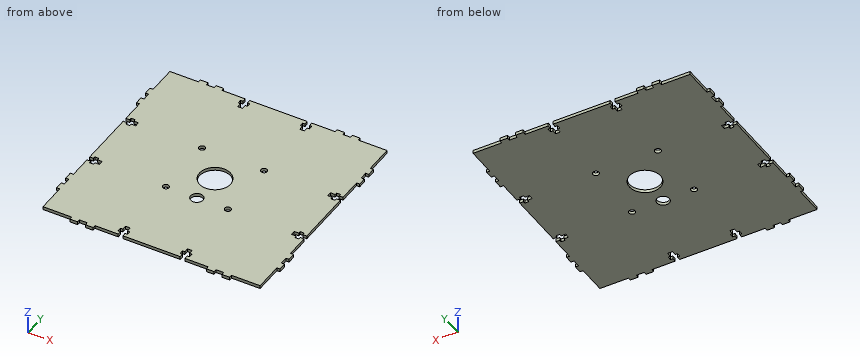
```python
from build123d import *

# Parameters (mm, degrees)
SKETCH_1_R      = 10
SKETCH_1_R_2    = 4
SKETCH_1_R_3    = 2
EXTRUDE_1_DEPTH = 2


with BuildPart() as part:
    # 草图1 → 凸台-拉伸1 (new body)
    with BuildSketch(Plane.XY):
        Polygon((317.453360513, 257.462931603), (317.453360513, 258.962931603), (314.853360513, 258.962931603), (314.853360513, 257.462931603), (311.853360513, 257.462931603), (311.853360513, 254.462931603), (314.853360513, 254.462931603), (314.853360513, 252.962931603), (317.453360513, 252.962931603), (317.453360513, 254.462931603), (319.953360513, 254.462931603), (319.953360513, 239.462931603), (321.953360513, 239.462931603), (321.953360513, 234.462931603), (319.953360513, 234.462931603), (319.953360513, 229.462931603), (321.953360513, 229.462931603), (321.953360513, 224.462931603), (319.953360513, 224.462931603), (319.953360513, 205.962931603), (301.453360513, 205.962931603), (301.453360513, 203.962931603), (296.453360513, 203.962931603), (296.453360513, 205.962931603), (291.453360513, 205.962931603), (291.453360513, 203.962931603), (286.453360513, 203.962931603), (286.453360513, 205.962931603), (271.453360513, 205.962931603), (271.453360513, 208.462931603), (272.953360513, 208.462931603), (272.953360513, 211.062931603), (271.453360513, 211.062931603), (271.453360513, 214.062931603), (268.453360513, 214.062931603), (268.453360513, 211.062931603), (266.953360513, 211.062931603), (266.953360513, 208.462931603), (268.453360513, 208.462931603), (268.453360513, 205.962931603), (231.453360513, 205.962931603), (231.453360513, 208.462931603), (232.953360513, 208.462931603), (232.953360513, 211.062931603), (231.453360513, 211.062931603), (231.453360513, 214.062931603), (228.453360513, 214.062931603), (228.453360513, 211.062931603), (226.953360513, 211.062931603), (226.953360513, 208.462931603), (228.453360513, 208.462931603), (228.453360513, 205.962931603), (213.453360513, 205.962931603), (213.453360513, 203.962931603), (208.453360513, 203.962931603), (208.453360513, 205.962931603), (203.453360513, 205.962931603), (203.453360513, 203.962931603), (198.453360513, 203.962931603), (198.453360513, 205.962931603), (179.953360513, 205.962931603), (179.953360513, 224.462931603), (177.953360513, 224.462931603), (177.953360513, 229.462931603), (179.953360513, 229.462931603), (179.953360513, 234.462931603), (177.953360513, 234.462931603), (177.953360513, 239.462931603), (179.953360513, 239.462931603), (179.953360513, 254.462931603), (182.453360513, 254.462931603), (182.453360513, 252.962931603), (185.053360513, 252.962931603), (185.053360513, 254.462931603), (188.053360513, 254.462931603), (188.053360513, 257.462931603), (185.053360513, 257.462931603), (185.053360513, 258.962931603), (182.453360513, 258.962931603), (182.453360513, 257.462931603), (179.953360513, 257.462931603), (179.953360513, 294.462931603), (182.453360513, 294.462931603), (182.453360513, 292.962931603), (185.053360513, 292.962931603), (185.053360513, 294.462931603), (188.053360513, 294.462931603), (188.053360513, 297.462931603), (185.053360513, 297.462931603), (185.053360513, 298.962931603), (182.453360513, 298.962931603), (182.453360513, 297.462931603), (179.953360513, 297.462931603), (179.953360513, 312.462931603), (177.953360513, 312.462931603), (177.953360513, 317.462931603), (179.953360513, 317.462931603), (179.953360513, 322.462931603), (177.953360513, 322.462931603), (177.953360513, 327.462931603), (179.953360513, 327.462931603), (179.953360513, 345.962931603), (198.453360513, 345.962931603), (198.453360513, 347.962931603), (203.453360513, 347.962931603), (203.453360513, 345.962931603), (208.453360513, 345.962931603), (208.453360513, 347.962931603), (213.453360513, 347.962931603), (213.453360513, 345.962931603), (228.453360513, 345.962931603), (228.453360513, 343.462931603), (226.953360513, 343.462931603), (226.953360513, 340.862931603), (228.453360513, 340.862931603), (228.453360513, 337.862931603), (231.453360513, 337.862931603), (231.453360513, 340.862931603), (232.953360513, 340.862931603), (232.953360513, 343.462931603), (231.453360513, 343.462931603), (231.453360513, 345.962931603), (268.453360513, 345.962931603), (268.453360513, 343.462931603), (266.953360513, 343.462931603), (266.953360513, 340.862931603), (268.453360513, 340.862931603), (268.453360513, 337.862931603), (271.453360513, 337.862931603), (271.453360513, 340.862931603), (272.953360513, 340.862931603), (272.953360513, 343.462931603), (271.453360513, 343.462931603), (271.453360513, 345.962931603), (286.453360513, 345.962931603), (286.453360513, 347.962931603), (291.453360513, 347.962931603), (291.453360513, 345.962931603), (296.453360513, 345.962931603), (296.453360513, 347.962931603), (301.453360513, 347.962931603), (301.453360513, 345.962931603), (319.953360513, 345.962931603), (319.953360513, 327.462931603), (321.953360513, 327.462931603), (321.953360513, 322.462931603), (319.953360513, 322.462931603), (319.953360513, 317.462931603), (321.953360513, 317.462931603), (321.953360513, 312.462931603), (319.953360513, 312.462931603), (319.953360513, 297.462931603), (317.453360513, 297.462931603), (317.453360513, 298.962931603), (314.853360513, 298.962931603), (314.853360513, 297.462931603), (311.853360513, 297.462931603), (311.853360513, 294.462931603), (314.853360513, 294.462931603), (314.853360513, 292.962931603), (317.453360513, 292.962931603), (317.453360513, 294.462931603), (319.953360513, 294.462931603), (319.953360513, 257.462931603), align=None)
        with Locations((249.953360513, 275.962931603)):
            Circle(SKETCH_1_R, mode=Mode.SUBTRACT)
        with Locations((249.953360513, 255.962931603)):
            Circle(SKETCH_1_R_2, mode=Mode.SUBTRACT)
        with Locations((229.953360513, 255.962931603)):
            Circle(SKETCH_1_R_3, mode=Mode.SUBTRACT)
        with Locations((229.953360513, 295.962931603)):
            Circle(SKETCH_1_R_3, mode=Mode.SUBTRACT)
        with Locations((269.953360513, 295.962931603)):
            Circle(SKETCH_1_R_3, mode=Mode.SUBTRACT)
        with Locations((269.953360513, 255.962931603)):
            Circle(SKETCH_1_R_3, mode=Mode.SUBTRACT)
    extrude(amount=EXTRUDE_1_DEPTH)


solid = part.part
```
Part model, mm, in its own coordinate system. Round coordinates to 2 decimals unless told otherwise and drop trailing zeros. Write each loop counter-clockwise with the first axis right and the second up, starting at its lowest first coordinate (ties: lowest second). Pieces come first, ordered by that corner, then holes. Notation, with made-up numbers: M 6.5,14.25 L 38.5,14.25 A11 cw 38.5,34.25 Z; hole C 50.25,-1 d9. An arc over 180 degrees is marked long. One line per question, with ' | ' between items.
(1) Pin check, flat tips, straight feed: pin 1 (0.6 mm diameter, centred on x = 316, z = 1, fed in from +Y); pin 2 (1 mm diameter, centred on x = 187, z = 1, fed in from -Y); pin 3 (0.6 mm diameter, centred on x = 178.5, z = 1.5, fed in from -Y). Stop position of each tip, or through.
Answer key:
pin 1: stops at y = 345.96 | pin 2: stops at y = 205.96 | pin 3: stops at y = 224.46
(2) Saw through at D-D on z = 1.3. Count the separate pieces of the cut face and the enclosed holes in it, then the cut area to 3 significant figures.
Answer key:
separate pieces: 1 | enclosed holes: 6 | area: 19,100 mm^2
(3) Probe line 1 along X through (y, z) = (340.5, 0.55); line 2 along Y through (x, z) = (251, 1.75); line 3 along Y through (x, z) = (271.5, 1.4). List the from-to ranges inside material, lowest first.
Answer key:
line 1: x = 179.95 to 228.45, 231.45 to 268.45, 271.45 to 319.95 | line 2: y = 205.96 to 252.1, 259.82 to 266.02, 285.91 to 345.96 | line 3: y = 205.96 to 208.46, 211.06 to 254.69, 257.23 to 294.69, 297.23 to 340.86, 343.46 to 345.96
(4) Saw through at A-A on y = 274. Write the cut outline in (x, z), then the cut area to 3 significant figures.
Answer key:
outline: M 179.95,0 L 240.15,0 L 240.15,2 L 179.95,2 Z; M 259.76,0 L 319.95,0 L 319.95,2 L 259.76,2 Z | area: 241 mm^2
(5) Saw through at B-B on x = 252. Write the cut outline in (y, z).
Answer key:
outline: M 205.96,0 L 252.53,0 L 252.53,2 L 205.96,2 Z; M 259.4,0 L 266.17,0 L 266.17,2 L 259.4,2 Z; M 285.75,0 L 345.96,0 L 345.96,2 L 285.75,2 Z
(6) Saw through at C-C on y = 247. Write the cut outline in (x, z), then the cut area to 3 significant figures.
Answer key:
outline: M 179.95,0 L 319.95,0 L 319.95,2 L 179.95,2 Z | area: 280 mm^2
